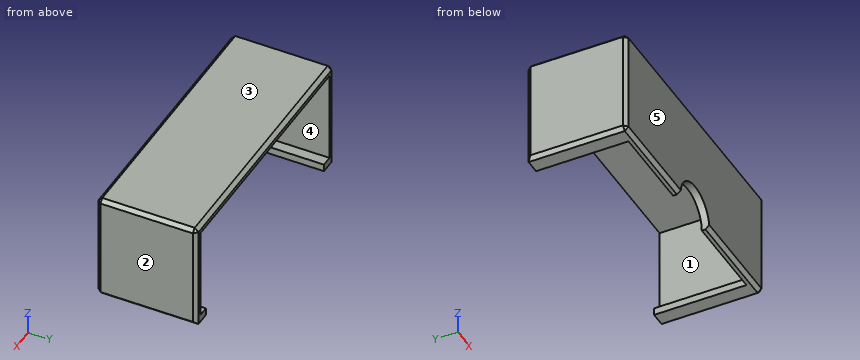
```python
from build123d import *

# Parameters (mm, degrees)
SKETCH1_W               = 71
SKETCH1_H               = 29
SKETCH1_W_2             = 67
SKETCH1_H_2             = 25
EXTRUDE_THIN1_DEPTH     = 24.7
CUT_EXTRUDE1_DEPTH      = 46.613484848
CUT_EXTRUDE1_DEPTH_BACK = 46.613484848
SKETCH2_W               = 61.246689818
SKETCH2_H               = 16.669960146
BOSS_EXTRUDE1_DEPTH     = 2
CHAMFER1_SIZE           = 1


with BuildPart() as part:
    # Sketch1 → Extrude-Thin1 (new body)
    with BuildSketch(Plane(origin=(0, 0, 0), x_dir=(1, 0, 0), z_dir=(0, 1, 0))):
        Rectangle(SKETCH1_W, SKETCH1_H)
        Rectangle(SKETCH1_W_2, SKETCH1_H_2, mode=Mode.SUBTRACT)
    extrude(amount=-EXTRUDE_THIN1_DEPTH)

    # Sketch2 → Cut-Extrude1 (cut, two sides: drawn at the far end of the back side and taken through both)
    with BuildSketch(Plane(origin=(0, 0, 0), x_dir=(1, 0, 0), z_dir=(0, 1, 0)).offset(-CUT_EXTRUDE1_DEPTH_BACK)):
        with Locations((0, 12.5)):
            Rectangle(SKETCH2_W, SKETCH2_H)
    extrude(amount=CUT_EXTRUDE1_DEPTH + CUT_EXTRUDE1_DEPTH_BACK, mode=Mode.SUBTRACT)

    # Sketch3 → Boss-Extrude1 (add)
    with BuildSketch(Plane.XZ.offset(24.7)):
        with BuildLine():
            Line((7.43, -14.5), (30.623344909, -14.5))
            Line((30.623344909, -14.5), (30.623344909, -12.5))
            Line((30.623344909, -12.5), (33.5, -12.5))
            Line((33.5, -12.5), (33.5, 12.5))
            Line((33.5, 12.5), (-33.5, 12.5))
            Line((-33.5, 12.5), (-33.5, -12.5))
            Line((-33.5, -12.5), (-30.623344909, -12.5))
            Line((-30.623344909, -12.5), (-30.623344909, -14.5))
            Line((-30.623344909, -14.5), (-7.43, -14.5))
            ThreePointArc((-7.43, -14.5), (0, -7.07), (7.43, -14.5))
        make_face()
        Polygon((33.5, 12.5), (33.5, -12.5), (30.623344909, -12.5), (30.623344909, -14.5), (35.5, -14.5), (35.5, 14.5), (-35.5, 14.5), (-35.5, -14.5), (-30.623344909, -14.5), (-30.623344909, -12.5), (-33.5, -12.5), (-33.5, 12.5), align=None)
    extrude(amount=BOSS_EXTRUDE1_DEPTH)

    # Chamfer1
    chamfer1_edges = [part.edges().sort_by_distance(p)[0] for p in [
        (0, 0, 14.5),
        (-35.5, 0, 0),
        (35.5, 0, 0),
        (21.465, -26.7, -14.5),
        (35.5, -26.7, 0),
        (0, -26.7, 14.5),
        (-35.5, -26.7, 0),
        (-21.465, -26.7, -14.5),
        (35.5, -13.35, 14.5),
        (-35.5, -13.35, 14.5),
        (-35.5, -13.35, -14.5),
        (35.5, -13.35, -14.5),
    ]]
    chamfer(chamfer1_edges, length=CHAMFER1_SIZE)


solid = part.part
```
Geometry check sheet. Reference: the model listing, model coordinates, mm. Face numbers are marked on the shaded views. A direction names the side the tool comes from. Give positions to 0.01 mm unless a question says otherwise; leave off trailing zeros. Loops run counter-clockwise (first coordinate to the right, second up) from the corner with the lowest first, then second, coordinate; pieces in that order, holes last. Notation, with made-up numbers: M 56.5,86.5 L 102.5,86.5 A20 ccw 102.5,106.5 Z; hole C 54,31 d3. An arc over 180 degrees is marked long. Write item = value, one per line. Start each with the question number.
1. Section check D-D, the plane z = 10.5. Enter the section's corners in (x, y), plus the area to 3 significant figures.
2. Go/stop test with flat-tipped pins: P1, Ø5, axis at x = 2, y = -12.5, coming from the -Z side; P2, Ø8, axis at x = -4.5, z = -0.5, coming from the +Y side. Record where each tip stops, or that it passes through.
3. Tool access check on the marked faces 1 and 2. Record the directions out of +Z, -Z, +X, -X, +Y, -Y that give a thin tool (end or side, any length) a straight path to the whole face; none if there is none.
4. Section check C-C, the plane y = -11. Enter the section's corners in (x, z), plus the area to 3 significant figures.
5. Draft check along Z on the marked faces 3, 4 and 5. Enter one of: +Z half, -Z half, draft (parallel to the pull), parting line (faces both ways), or undercut.
6. Thickness scan on probe 1 along X at (y, z) = (-7, 4.5); probe 2 along X at (y, z) = (-9.5, -12.75); probe 3 along Y at (x, z) = (-19.5, 6.5). Record the ranges inside material, lowest first.
7. Section check A-A, the plane x = 0. Enter the section's corners in (y, z).
8. Section check B-B, the plane z = -11.5. Enter the section's corners in (x, y), plus the area to 3 significant figures.
Values follow:
q1.outline = M -35.5,-25.7 L -34.5,-26.7 L 34.5,-26.7 L 35.5,-25.7 L 35.5,-1 L 34.5,0 L 33.5,0 L 33.5,-24.7 L -33.5,-24.7 L -33.5,0 L -34.5,0 L -35.5,-1 Z
q1.area = 239 mm^2
q2.P1 = 12.5
q2.P2 = -24.7
q3.face_1 = +Y
q3.face_2 = +Z, -Z, +X, +Y, -Y
q4.outline = M -35.5,-13.5 L -34.5,-14.5 L -30.62,-14.5 L -30.62,-12.5 L -33.5,-12.5 L -33.5,12.5 L 33.5,12.5 L 33.5,-12.5 L 30.62,-12.5 L 30.62,-14.5 L 34.5,-14.5 L 35.5,-13.5 L 35.5,13.5 L 34.5,14.5 L -34.5,14.5 L -35.5,13.5 Z
q4.area = 260 mm^2
q5.face_3 = +Z half
q5.face_4 = undercut
q5.face_5 = draft
q6.probe_1 = -35.5 to -33.5, 33.5 to 35.5
q6.probe_2 = -35.5 to -30.62, 30.62 to 35.5
q6.probe_3 = -26.7 to -24.7
q7.outline = M -26.7,-7.07 L -24.7,-7.07 L -24.7,12.5 L 0,12.5 L 0,13.5 L -1,14.5 L -25.7,14.5 L -26.7,13.5 Z
q8.outline = M -35.5,-25.7 L -34.5,-26.7 L -6.8,-26.7 L -6.8,-24.7 L -33.5,-24.7 L -33.5,0 L -34.5,0 L -35.5,-1 Z; M 6.8,-26.7 L 34.5,-26.7 L 35.5,-25.7 L 35.5,-1 L 34.5,0 L 33.5,0 L 33.5,-24.7 L 6.8,-24.7 Z
q8.area = 212 mm^2
